```python
from build123d import *

# Parameters (mm, degrees)
SKETCH1_R           = 1.75
BOSS_EXTRUDE1_DEPTH = 6
SKETCH1_3_W         = 90
SKETCH1_3_H         = 59.090909091
BOSS_EXTRUDE2_DEPTH = 85


with BuildPart() as part:
    # Sketch1 → Boss-Extrude1 (new body)
    with BuildSketch(Plane(origin=(0, 0, 0), x_dir=(1, 0, 0), z_dir=(0, 1, 0))):
        Polygon((-35, 27.5), (-35, 32.5), (-55, 32.5), (-55, -32.5), (-45, -32.5), (-45, 26.590909091), (45, 26.590909091), (45, -32.5), (55, -32.5), (55, 32.5), (35, 32.5), (35, 27.5), (15, 27.5), (15, 32.5), (-15, 32.5), (-15, 27.5), align=None)
        with Locations(Location((-50, -22.5, 0), (0, 0, 270))):
            Circle(SKETCH1_R, mode=Mode.SUBTRACT)
        with Locations(Location((50, -22.5, 0), (0, 0, 270))):
            Circle(SKETCH1_R, mode=Mode.SUBTRACT)
        with Locations(Location((-50, 17.5, 0), (0, 0, 270))):
            Circle(SKETCH1_R, mode=Mode.SUBTRACT)
        with Locations(Location((50, 17.5, 0), (0, 0, 270))):
            Circle(SKETCH1_R, mode=Mode.SUBTRACT)
    extrude(amount=BOSS_EXTRUDE1_DEPTH)

    # Sketch1_3 → Boss-Extrude2 (add)
    with BuildSketch(Plane(origin=(0, 0, 0), x_dir=(1, 0, 0), z_dir=(0, 1, 0))):
        with Locations((0, -2.954545454)):
            Rectangle(SKETCH1_3_W, SKETCH1_3_H)
    extrude(amount=BOSS_EXTRUDE2_DEPTH)


solid = part.part
```
The listing builds one solid part. Answer for the finished solid, in the listing's coordinates (mm). A direction names the side the tool comes from. Coordinates: 2 decimals unless noted, no trailing zeros. Loops run counter-clockwise (first coordinate to the right, second up) from the corner with the lowest first, then second, coordinate; pieces in that order, holes last. Notation, with made-up numbers: M 52.25,40.5 L 104.25,40.5 A28 ccw 104.25,72.5 Z; hole C 44,-8 d6. An arc over 180 degrees is marked long. Answer as a JSON object with one key per item and string values. Group by question number.
Item 1: Section B-B (x = 50) is taken. Write down the section's boundary in (y, z).
Item 2: Section C-C (z = 14) is taken. Write down the section's boundary in (x, y), and give its area (3 significant figures).
Item 3: Each of these flat-tipped pins is pushed along its axis until it touches: P1, Ø1, axis at y = 20.5, z = 17.5, coming from the +X side; P2, Ø17.5, axis at y = 35, z = 1, coming from the -X side; P3, Ø5, axis at x = 28.5, y = 4, coming from the -Z side. Where does it stop, or does it pass through?
Item 4: Section A-A (z = 22.5) is taken. Write down the section's boundary in (x, y), and give its area (3 significant figures).
Item 5: Which of the six approach directions +Z, -Z, +X, -X, +Y, -Y give full straight-line access (tool end or side, diameter ignored) to faces 1 (the face through (45, 45, 3)), 2 (the face through (-15, 3, -30)), 3 (the face through (-51.06, 2.96, 21.11)), 4 (the face through (-45, 45, 3)), 5 (the face through (45, 3, -32.5))?
Item 6: Section D-D (x = 13) is taken. Write down the section's boundary in (y, z), and give its area (3 significant figures).
Item 7: Consider L1, parallel to X at y = 3.95, z = -17.5; L2, parallel to X at y = 5.5, z = -29; L3, parallel to Z at x = 40, y = 11. Determine where each line is inside the solid, lowest interval first.
Item 8: Determine the mould class of faces 6 (the face through (-25, 3, -27.5)), 7 (the face through (48.29, 2.96, -17.88)), 8 (the face through (55, 3, 0)) for opening direction Z: +Z half, -Z half, draft (parallel to the pull), parting line (faces both ways), or undercut.
Solved:
{
 "1": {"outline": "M 0,-32.5 L 6,-32.5 L 6,-19.25 L 0,-19.25 Z; M 0,-15.75 L 6,-15.75 L 6,20.75 L 0,20.75 Z; M 0,24.25 L 6,24.25 L 6,32.5 L 0,32.5 Z"},
 "2": {"outline": "M -55,0 L 55,0 L 55,6 L 45,6 L 45,85 L -45,85 L -45,6 L -55,6 Z", "area": "7,770 mm2"},
 "3": {"P1": "stops at x = 45", "P2": "stops at x = -45", "P3": "stops at z = -27.5"},
 "4": {"outline": "M -55,0 L -51.75,0 L -51.75,6 L -55,6 Z; M -48.25,0 L 48.25,0 L 48.25,6 L 45,6 L 45,85 L -45,85 L -45,6 L -48.25,6 Z; M 51.75,0 L 55,0 L 55,6 L 51.75,6 Z", "area": "7,730 mm2"},
 "5": {"face 1": "+Z, -Z, +X, +Y", "face 2": "-Z, +Y, -Y", "face 3": "+Y, -Y", "face 4": "+Z, -Z, -X, +Y", "face 5": "-Z, +X, -X, +Y, -Y"},
 "6": {"outline": "M 0,-32.5 L 6,-32.5 L 6,-26.59 L 85,-26.59 L 85,32.5 L 0,32.5 Z", "area": "5,060 mm2"},
 "7": {"L1": "x = -55 to -51.75, -48.25 to 48.25, 51.75 to 55", "L2": "x = -55 to -35, -15 to 15, 35 to 55", "L3": "z = -26.59 to 32.5"},
 "8": {"face 6": "-Z half", "face 7": "undercut", "face 8": "draft"}
}
